Check sheet for the modelled part. Datum: model origin and axes. Units: mm. Face numbers are marked on the shaded views. A direction names the side the tool comes from. Round coordinates to 2 decimals unless told otherwise and drop trailing zeros. Write each loop counter-clockwise with the first axis right and the second up, starting at its lowest first coordinate (ties: lowest second). Pieces come first, ordered by that corner, then holes.
Item 1: Section check C-C, the plane x = 28. Record the cut outline in (y, z).
Item 2: Set-up check for the marked faces 1, 2 and 3: record each of +Z, -Z, +X, -X, +Y, -Y from which the full face is reachable in a straight line by a thin tool's end or side.
Item 3: Section check A-A, the plane z = 19.5. Record the cut outline in (x, y), plus the area to 3 significant figures.
Item 4: Material ranges on line 1 along Y through (x, z) = (46, 8); line 2 along X through (y, z) = (10, 30); line 3 along X through (y, z) = (-5, 24.5), recorded low to high.
Item 5: Section check D-D, the plane x = 41.5. Record the cut outline in (y, z).
Item 6: Depth check by flat-ended pin: pin 1 (12 mm diameter, centred on x = 36, z = 4.5, fed in from +Y); pin 2 (10 mm diameter, centred on x = 36.5, z = 13, fed in from -Y); pin 3 (9.5 mm diameter, centred on x = 33, z = 17.5, fed in from +Y). Enter the tip coordinate at first touch or a pass-through.
Item 7: Section check B-B, the plane y = -6.5. Record the cut outline in (x, z).
from build123d import *

# Parameters (mm, degrees)
F1_DEPTH = 25.4
F3_DEPTH = 38.1
F5_DEPTH = 12.7
F6_DEPTH = 12.7
F8_DEPTH = 12.7


# Not quite as in the source:
# - a length typed as a fraction of an inch, garbled in the dataset ("3 / 203.2 mm" for 3/8 in), is restored


with BuildPart() as f1:
    # F0 (on Front) → F1 (new body)
    with BuildSketch(Plane.XZ):
        Polygon((57.15, 31.7493037554), (0, 31.7493037554), (0, 0), (56.9397357658, 0), align=None)
    extrude(amount=F1_DEPTH)

    # F2 (on face) → F3 (cut)
    with BuildSketch(Plane.XZ.offset(25.4)):
        Polygon((44.45, 31.7493037554), (56.9397357658, 0), (57.15, 31.7493037554), align=None)
    extrude(amount=-F3_DEPTH, mode=Mode.SUBTRACT)

    # F4 (on face) → F5 (cut)
    with BuildSketch(Plane.XZ.offset(25.4)):
        Polygon((44.45, 31.7493037554), (19.05, 31.7493037554), (31.5397357658, 0), (56.9397357658, 0), align=None)
    extrude(amount=-F5_DEPTH, mode=Mode.SUBTRACT)

    # F6 (add): a face of the model
    f6_faces = [f1.faces().sort_by_distance(p)[0] for p in [
        (25.4756467057, 0, 15.2228100654),
    ]]
    extrude(f6_faces, amount=F6_DEPTH)

    # F7 (on face) → F8 (cut)
    with BuildSketch(Plane(origin=(0, 12.7, 0), x_dir=(-1, 0, 0), z_dir=(0, 1, 0))):
        Polygon((-56.9397357658, 0), (-31.5397357658, 0), (-19.05, 31.7493037554), (-44.45, 31.7493037554), align=None)
    extrude(amount=-F8_DEPTH, mode=Mode.SUBTRACT)


solid = f1.part
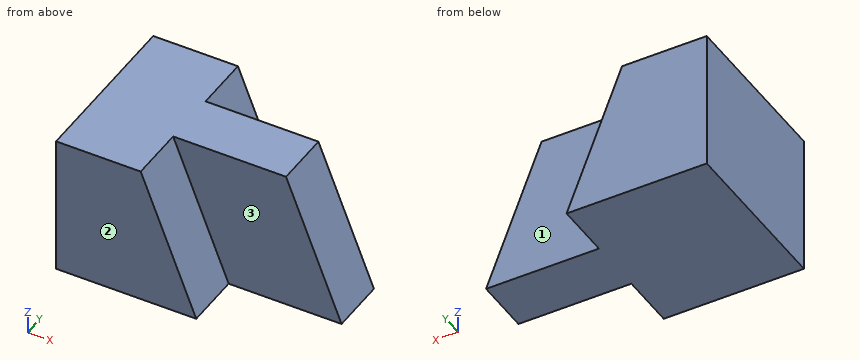
Values found:
1. outline: (-25.4, 0) - (12.7, 0) - (12.7, 9) - (0, 9) - (0, 31.75) - (-12.7, 31.75) - (-12.7, 9) - (-25.4, 9) - close
2. face 1: +Z, +X, +Y
2. face 2: +Z, -Z, +X, -X, -Y
2. face 3: +Z, +X, -Y
3. outline: (0, -25.4) - (23.87, -25.4) - (23.87, -12.7) - (49.27, -12.7) - (49.27, 0) - (23.87, 0) - (23.87, 12.7) - (0, 12.7) - close
3. area: 1,230 mm2
4. line 1: y = -12.7 to 0
4. line 2: x = 0 to 19.74
4. line 3: x = 0 to 47.3
5. outline: (-12.7, 0) - (0, 0) - (0, 31.75) - (-12.7, 31.75) - close
6. pin 1: stops at y = 12.7
6. pin 2: stops at y = -12.7
6. pin 3: stops at y = 0
7. outline: (0, 0) - (56.94, 0) - (44.45, 31.75) - (0, 31.75) - close
